from build123d import *

# Parameters (mm, degrees)
BOSS_EXTRUDE1_DEPTH = 1
SKETCH2_R           = 15
CUT_EXTRUDE1_DEPTH  = 10


with BuildPart() as part:
    # Sketch1 → Boss-Extrude1 (new body)
    with BuildSketch(Plane.XY):
        Polygon((-48, 40.5), (-40.5, 40.5), (-40.5, 48), (40.5, 48), (40.5, 40.5), (48, 40.5), (48, -40.5), (40.5, -40.5), (40.5, -48), (-40.5, -48), (-40.5, -40.5), (-48, -40.5), align=None)
    extrude(amount=BOSS_EXTRUDE1_DEPTH)

    # Sketch2 → Cut-Extrude1 (cut)
    with BuildSketch(Plane.XY.offset(1)):
        Circle(SKETCH2_R)
    extrude(amount=-CUT_EXTRUDE1_DEPTH, mode=Mode.SUBTRACT)


solid = part.part
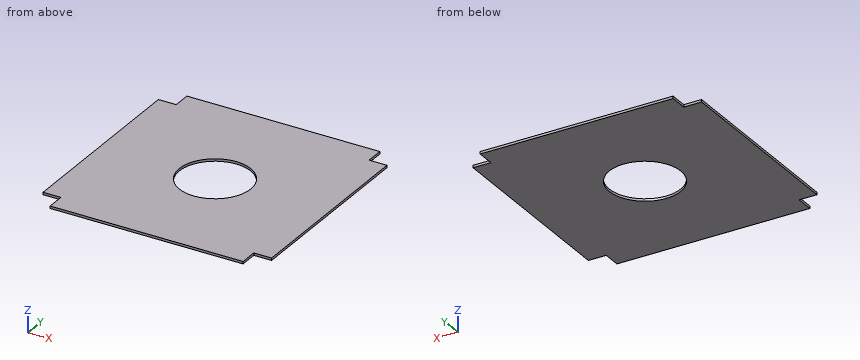
The listing builds one solid part. Answer for the finished solid, in the listing's coordinates (mm). Coordinates: 2 decimals unless noted, no trailing zeros. Order: outer loops, then holes, each group sorted by start corner. A loop starts at its lowest first (then second) coordinate and runs counter-clockwise, first axis right, second up.
Q1. Consider line 1 (Y direction, x = 0, z = 0.5); line 2 (Y direction, x = -9.5, z = 0.15); line 3 (X direction, y = -8, z = 0.75). Determine where each line is inside the solid, lowest interval first.
Q2. A cutting plane is placed at B-B, the plane x = 0. Write down the section's boundary in (y, z).
Q3. Given P1, Ø0.5, axis at y = -46, z = 0.5, coming from the -X side; P2, Ø0.5, axis at x = 43, z = 0.5, coming from the +Y side; P3, Ø0.5, axis at y = 44, z = 0.5, coming from the +X side; P4, Ø1, axis at x = 8.5, y = -10.5, coming from the -Z side, each flat-ended and moving along its own axis, determine where each tip first touches the part or whether it passes through.
Q4. A cutting plane is placed at A-A, the plane z = 0.3. Write down the section's boundary in (x, y), and give its area (3 significant figures).
Q5. A cutting plane is placed at C-C, the plane y = -5. Write down the section's boundary in (x, z), and give its area (3 significant figures).
Answers follow:
1. line 1: y = -48 to -15, 15 to 48
1. line 2: y = -48 to -11.61, 11.61 to 48
1. line 3: x = -48 to -12.69, 12.69 to 48
2. outline: (-48, 0) - (-15, 0) - (-15, 1) - (-48, 1) - close; (15, 0) - (48, 0) - (48, 1) - (15, 1) - close
3. P1: stops at x = -40.5
3. P2: stops at y = 40.5
3. P3: stops at x = 40.5
3. P4: passes through
4. outline: (-48, -40.5) - (-40.5, -40.5) - (-40.5, -48) - (40.5, -48) - (40.5, -40.5) - (48, -40.5) - (48, 40.5) - (40.5, 40.5) - (40.5, 48) - (-40.5, 48) - (-40.5, 40.5) - (-48, 40.5) - close; hole circle Ø30 at (0, 0)
4. area: 8,280 mm2
5. outline: (-48, 0) - (-14.14, 0) - (-14.14, 1) - (-48, 1) - close; (14.14, 0) - (48, 0) - (48, 1) - (14.14, 1) - close
5. area: 67.7 mm2
